Verification items for the finished model (mm, model axes). Face numbers are marked on the shaded views. A direction names the side the tool comes from. Give positions to 0.01 mm unless a question says otherwise; leave off trailing zeros. Loops run counter-clockwise (first coordinate to the right, second up) from the corner with the lowest first, then second, coordinate; pieces in that order, holes last. Notation, with made-up numbers: M 64,53.25 L 115,53.25 A25 cw 115,72.25 Z; hole C -19,35 d5. An arc over 180 degrees is marked long. Use a Markdown table: item, result.
from build123d import *

# Parameters (mm, degrees)
F0_R     = 3.1
F1_DEPTH = 10
F2_DEPTH = 1.5
F3_W     = 20
F3_H     = 2
F4_DEPTH = 11.501


# Not quite as in the source:
# - a feature names something its author has since deleted; it is built from what else it names


with BuildPart() as f1:
    # F0 (on Top) → F1 (new body, symmetric)
    with BuildSketch(Plane.XY):
        Circle(F0_R)
    extrude(amount=F1_DEPTH, both=True)

    # F0 (on Top) → F2 (join, symmetric)
    with BuildSketch(Plane.XY):
        with BuildLine():
            ThreePointArc((0.9128866521, -9.9582447229), (7.3867742121, -6.7405909785), (10, 0))
            ThreePointArc((10, 0), (7.3867742121, 6.7405909785), (0.9128866521, 9.9582447229))
            ThreePointArc((0.9128866521, 9.9582447229), (-10, 0), (0.9128866521, -9.9582447229))
        make_face()
        Circle(F0_R, mode=Mode.SUBTRACT)
        with BuildLine():
            ThreePointArc((0.9128866521, 9.9582447229), (7.3867742121, 6.7405909785), (10, 0))
            ThreePointArc((10, 0), (7.3867742121, -6.7405909785), (0.9128866521, -9.9582447229))
            Line((0.9128866521, -9.9582447229), (55, -5))
            Line((55, -5), (55, 5))
            Line((55, 5), (0.9128866521, 9.9582447229))
        make_face()
    extrude(amount=F2_DEPTH, both=True)

    # F3 (on face) → F4 (cut, through all)
    with BuildSketch(Plane.XY.offset(1.5)):
        with Locations((45, 0)):
            Rectangle(F3_W, F3_H)
    extrude(amount=-F4_DEPTH, mode=Mode.SUBTRACT)


solid = f1.part
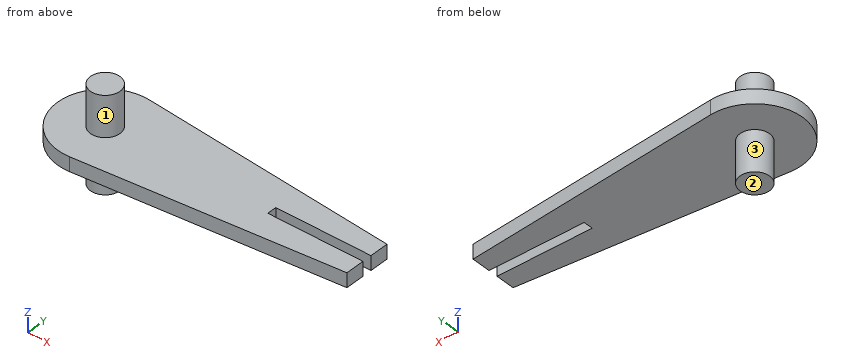
(1) Cross-section at C-C on x = 0. Record the cut outline in (y, z).
Results below:
| item | result |
|---|---|
| outline | M -10,-1.5 L -3.1,-1.5 L -3.1,-10 L 3.1,-10 L 3.1,-1.5 L 10,-1.5 L 10,1.5 L 3.1,1.5 L 3.1,10 L -3.1,10 L -3.1,1.5 L -10,1.5 Z |
(2) Gauge pin test, flat ends, axial feed: P1, Ø3, axis at x = 34, y = -6, coming from the -Z side; P2, Ø5, axis at x = 12.5, z = 2, coming from the -Y side; P3, Ø5, axis at x = 47.5, y = -3.5, coming from the +Z side. Record the tip position at first contact, or that the pin passes through.
Results below:
| item | result |
|---|---|
| P1 | z = -1.5 |
| P2 | y = -9.12 |
| P3 | z = 1.5 |
(3) Material ranges on line 1 (Z direction, x = 25, y = -3.75); line 2 (X direction, y = -1.5, z = -7); line 3 (Y direction, x = 43, z = -1.25), recorded low to high.
Results below:
| item | result |
|---|---|
| line 1 | -1.5 to 1.5 |
| line 2 | -2.71 to 2.71 |
| line 3 | -6.1 to -1, 1 to 6.1 |
(4) Cross-section at B-B on y = 0. Record the cut outline in (x, z), then the cut area to 3 significant figures.
Results below:
| item | result |
|---|---|
| outline | M -10,-1.5 L -3.1,-1.5 L -3.1,-10 L 3.1,-10 L 3.1,-1.5 L 35,-1.5 L 35,1.5 L 3.1,1.5 L 3.1,10 L -3.1,10 L -3.1,1.5 L -10,1.5 Z |
| area | 240 mm^2 |
(5) Set-up check for the marked faces 1, 2 and 3: record each of +Z, -Z, +X, -X, +Y, -Y from which the full face is reachable in a straight line by a thin tool's end or side.
Results below:
| item | result |
|---|---|
| face 1 | +Z |
| face 2 | -Z, +X, -X, +Y, -Y |
| face 3 | -Z |
(6) Cross-section at D-D on z = 4. Record the cut outline in (x, y).
Results below:
| item | result |
|---|---|
| outline | C 0,0 d6.2 |
(7) Cross-section at A-A on x = 39.5. Record the cut outline in (y, z).
Results below:
| item | result |
|---|---|
| outline | M -6.42,-1.5 L -1,-1.5 L -1,1.5 L -6.42,1.5 Z; M 1,-1.5 L 6.42,-1.5 L 6.42,1.5 L 1,1.5 Z |
